Verification items for the finished model (mm, model axes). Face numbers are marked on the shaded views. Give positions to 0.01 mm unless a question says otherwise; leave off trailing zeros. Write each loop counter-clockwise with the first axis right and the second up, starting at its lowest first coordinate (ties: lowest second). Pieces come first, ordered by that corner, then holes. Notation, with made-up numbers: M 72,45 L 114,45 A22 ccw 114,55 Z; hole C 16,7.25 d1. An arc over 180 degrees is marked long. Write item = value, one per line.
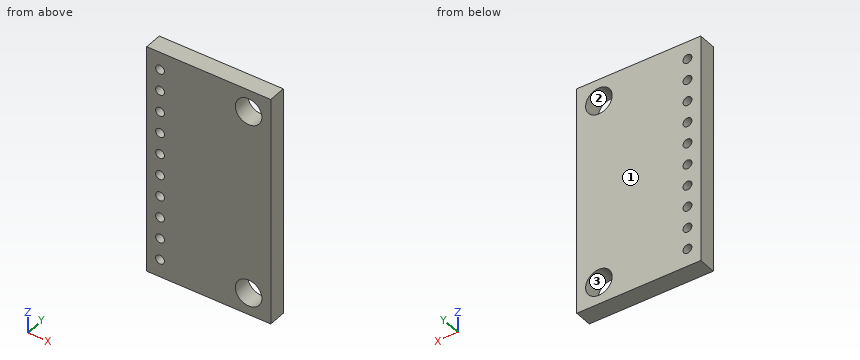
from build123d import *

# Parameters (mm, degrees)
SKETCH1_W           = 14
SKETCH1_H           = 26
BOSS_EXTRUDE1_DEPTH = 2
SKETCH2_R           = 1.5
CUT_EXTRUDE1_DEPTH  = 15.899664426
SKETCH3_R           = 0.5
CUT_EXTRUDE2_DEPTH  = 15.899664426


with BuildPart() as part:
    # Sketch1 → Boss-Extrude1 (new body)
    with BuildSketch(Plane(origin=(0, 0, 0), x_dir=(1, 0, 0), z_dir=(0, 1, 0))):
        Rectangle(SKETCH1_W, SKETCH1_H)
    extrude(amount=BOSS_EXTRUDE1_DEPTH)

    # Sketch2 → Cut-Extrude1 (cut, through all)
    with BuildSketch(Plane(origin=(0, 2, 0), x_dir=(1, 0, 0), z_dir=(0, 1, 0))):
        with Locations(Location((4.5, 10.5, 0), (0, 0, 270))):
            Circle(SKETCH2_R)
        with Locations(Location((4.5, -10.5, 0), (0, 0, 270))):
            Circle(SKETCH2_R)
    extrude(amount=-CUT_EXTRUDE1_DEPTH, mode=Mode.SUBTRACT)

    # Sketch3 → Cut-Extrude2 (cut, through all)
    with BuildSketch(Plane(origin=(0, 2, 0), x_dir=(1, 0, 0), z_dir=(0, 1, 0))):
        with Locations(Location((-5.5, 11, 0), (0, 0, 270))):
            Circle(SKETCH3_R)
        with Locations(Location((-5.5, 8.555556, 0), (0, 0, 270))):
            Circle(SKETCH3_R)
        with Locations(Location((-5.5, 6.111112, 0), (0, 0, 270))):
            Circle(SKETCH3_R)
        with Locations(Location((-5.5, 3.666668, 0), (0, 0, 270))):
            Circle(SKETCH3_R)
        with Locations(Location((-5.5, 1.222224, 0), (0, 0, 270))):
            Circle(SKETCH3_R)
        with Locations(Location((-5.5, -1.22222, 0), (0, 0, 270))):
            Circle(SKETCH3_R)
        with Locations(Location((-5.5, -3.666664, 0), (0, 0, 270))):
            Circle(SKETCH3_R)
        with Locations(Location((-5.5, -6.111108, 0), (0, 0, 270))):
            Circle(SKETCH3_R)
        with Locations(Location((-5.5, -8.555552, 0), (0, 0, 270))):
            Circle(SKETCH3_R)
        with Locations(Location((-5.5, -10.999996, 0), (0, 0, 270))):
            Circle(SKETCH3_R)
    extrude(amount=-CUT_EXTRUDE2_DEPTH, mode=Mode.SUBTRACT)


solid = part.part
1) Material ranges on probe 1 along X at (y, z) = (0.4, -1); probe 2 along Z at (x, y) = (5.5, 0.5); probe 3 along X at (y, z) = (0.75, -3.5), recorded low to high. Write a range as from..to.
From the geometry:
probe_1 = -7..-5.95, -5.05..7
probe_2 = -13..-11.62, -9.38..9.38, 11.62..13
probe_3 = -7..-5.97, -5.03..7
2) Cross-section at B-B on x = 4.5. Record the boundary of the cut face in (y, z), plus the area to 3 significant figures.
From the geometry:
outline = M 0,-13 L 2,-13 L 2,-12 L 0,-12 Z; M 0,-9 L 2,-9 L 2,9 L 0,9 Z; M 0,12 L 2,12 L 2,13 L 0,13 Z
area = 40.0 mm^2
3) Cross-section at C-C on z = -11. Record the boundary of the cut face in (x, y), plus the area to 3 significant figures.
From the geometry:
outline = M -7,0 L -6,0 L -6,2 L -7,2 Z; M -5,0 L 3.09,0 L 3.09,2 L -5,2 Z; M 5.91,0 L 7,0 L 7,2 L 5.91,2 Z
area = 20.3 mm^2
4) Cross-section at A-A on y = 1.3. Count the separate pieces of the cut face and the enclosed holes in it, plus the area to 3 significant figures.
From the geometry:
separate_pieces = 1
enclosed_holes = 12
area = 342 mm^2
5) Draft check along Z on the marked faces 1, 2 and 3. Enter one of: +Z half, -Z half, draft (parallel to the pull), parting line (faces both ways), or undercut.
From the geometry:
face_1 = draft
face_2 = undercut
face_3 = undercut
